For this review, take the finished solid that the model builds, in its own axes (mm). A direction names the side the tool comes from. Round coordinates to 2 decimals unless told otherwise and drop trailing zeros. Order: outer loops, then holes, each group sorted by start corner. A loop starts at its lowest first (then second) coordinate and runs counter-clockwise, first axis right, second up. Notation, with made-up numbers: M -15.5,-19 L -2.5,-19 A20 ccw -2.5,-2 Z; hole C 48,77.5 d6. An arc over 180 degrees is marked long. Use a Markdown table: item, result.
from build123d import *

# Parameters (mm, degrees)
F0_W     = 6
F0_H     = 3
F1_DEPTH = 5
F2_R     = 1.5
F3_DEPTH = 100
F4_DEPTH = 100


with BuildPart() as f1:
    # F0 (on Front) → F1 (new body)
    with BuildSketch(Plane.XZ):
        with Locations((-12.822277, 42.440869)):
            Rectangle(F0_W, F0_H)
        Polygon((28.177723, 30.940869), (-9.822277, 43.940869), (-9.822277, 40.940869), (28.177723, 27.940869), align=None)
        with Locations((31.177723, 29.440869)):
            Rectangle(F0_W, F0_H)
    extrude(amount=F1_DEPTH)

    # F2 (on Top) → F3 (cut)
    with BuildSketch(Plane.XY):
        with Locations((-12.822277, -2.5)):
            Circle(F2_R)
    extrude(amount=F3_DEPTH, mode=Mode.SUBTRACT)

    # F2 (on Top) → F4 (cut)
    with BuildSketch(Plane.XY):
        with Locations((-12.822277, -2.5)):
            Circle(F2_R)
        with Locations((31.177723, -2.5)):
            Circle(F2_R)
    extrude(amount=F4_DEPTH, mode=Mode.SUBTRACT)


solid = f1.part
Q1. Clearance check with flat-ended pins moving along their axes: pin 1 (2 mm diameter, centred on x = 10, y = -3.5, fed in from +Z); pin 2 (2.5 mm diameter, centred on x = 31.18, y = -2.5, fed in from -Z). State where each tip first meets the part, or that it passes through.
Determined:
| item | result |
|---|---|
| pin 1 | stops at z = 37.5 |
| pin 2 | passes through |
Q2. Add section B-B (x = -8). Write out the cut boundary in (y, z).
Determined:
| item | result |
|---|---|
| outline | M -5,40.32 L 0,40.32 L 0,43.32 L -5,43.32 Z |
Q3. Add section A-A (y = -2.5). Write out the cut boundary in (x, z).
Determined:
| item | result |
|---|---|
| outline | M -15.82,40.94 L -14.32,40.94 L -14.32,43.94 L -15.82,43.94 Z; M -11.32,40.94 L -9.82,40.94 L 28.18,27.94 L 29.68,27.94 L 29.68,30.94 L 28.18,30.94 L -9.82,43.94 L -11.32,43.94 Z; M 32.68,27.94 L 34.18,27.94 L 34.18,30.94 L 32.68,30.94 Z |
Q4. Machinability: for faces 1 (the flat face through (34.178, -2, 29)), 2 (the flat face through (31.1, -0.8, 30.941)), which of the approach directions +Z, -Z, +X, -X, +Y, -Y give a long, thin tool a straight path to every point of the face, cutting with its end or side? Answer none if there is none.
Determined:
| item | result |
|---|---|
| face 1 | +Z, -Z, +X, +Y, -Y |
| face 2 | +Z, +X, +Y, -Y |
Q5. Add section C-C (z = 40.5). Write out the cut boundary in (x, y), then the cut area to 3 significant figures.
Determined:
| item | result |
|---|---|
| outline | M -8.53,-5 L 0.24,-5 L 0.24,0 L -8.53,0 Z |
| area | 43.8 mm^2 |
Q6. Draft analysis for pull direction X (two halves, no side actions). For faces 3 (the flat face through (-12.9, -0.8, 40.941)), 4 (the cylindrical face through (32.61, -2.05, 29.42)), 5 (the flat face through (-15.822, -2, 42)), 6 (the cylindrical face through (-11.39, -2.05, 42.42)), state which applies: pulls with the +X half, pulls with the -X half, needs draft (parallel to the pull), parting line crosses it, or undercut.
Determined:
| item | result |
|---|---|
| face 3 | needs draft |
| face 4 | undercut |
| face 5 | pulls with the -X half |
| face 6 | undercut |
Q7. Wall thickness on line 1 along Z through (x, y) = (-11.5, -0.8); line 2 along Z through (x, y) = (31.5, -0.7): over which ranges is each line inside the solid? List them lowest first. Write a range as [from, to].
Determined:
| item | result |
|---|---|
| line 1 | z = [40.94, 43.94] |
| line 2 | z = [27.94, 30.94] |
